Design review of the part shown in the three views and the two pictorial views. Dimensions are in mm from the part's minimum x, y and z. Round coordinates to 2 decimals unless told otherwise and drop trailing zeros. Loops run counter-clockwise (first coordinate to the right, second up) from the corner with the lowest first, then second, coordinate; pieces in that order, holes last. Notation, with made-up numbers: (59.5, -4.5) -> (107.5, -4.5) arc R24 ccw to (107.5, 20.5) -> close; hole circle Ø8 at (14.25, 87). An arc over 180 degrees is marked (long way). Use a Markdown table: item, result. Add a question column.
1) Consider section A-A on x = 2.85. Give the boundary of the cut face in (y, z).
2) Consider section B-B on z = 15.5. Give the boundary of the cut face in (x, y), plus the area to 3 significant figures.
3) Wall thickness on probe 1 along Z at (x, y) = (2, 4.65); probe 2 along Y at (x, z) = (2.95, 10.5); probe 3 along Y at (x, z) = (4.95, 31): over which ranges is each line inside the solid? List them lowest first.
4) Consider section C-C on y = 3.75. Give the boundary of the cut face in (x, z).
5) Mouldability with a two-part tool opening along Z and no side actions: class the marked faces 1, 2 and 3 as released by +Z, released by -Z, zero draft, split by the parting line, or undercut.
6) Insertion check: pin 1 (0.6 mm diameter, centred on x = 2.5, z = 16, fed in from -Y); pin 2 (3 mm diameter, centred on x = 4.5, z = 17, fed in from +Y); pin 3 (2 mm diameter, centred on x = 1.5, z = 30.5, fed in from -Y). Each pin has a flat end and moves straight along its axis. Give the tip position at first contact, or say it passes through.
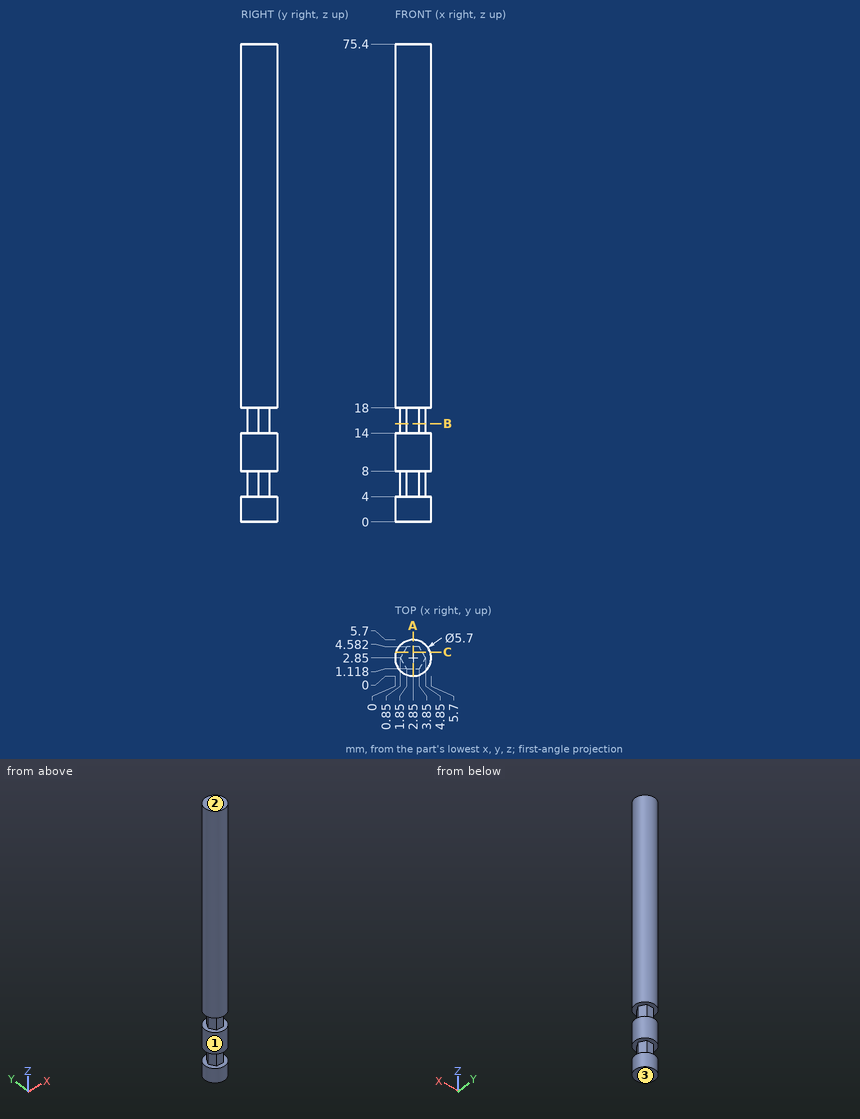
Result set:
| question | item | result |
|---|---|---|
| 1 | outline | (0, 0) -> (5.7, 0) -> (5.7, 4) -> (4.58, 4) -> (4.58, 8) -> (5.7, 8) -> (5.7, 14) -> (4.58, 14) -> (4.58, 18) -> (5.7, 18) -> (5.7, 75.4) -> (0, 75.4) -> (0, 18) -> (1.12, 18) -> (1.12, 14) -> (0, 14) -> (0, 8) -> (1.12, 8) -> (1.12, 4) -> (0, 4) -> close |
| 2 | outline | (0.85, 2.85) -> (1.85, 1.12) -> (3.85, 1.12) -> (4.85, 2.85) -> (3.85, 4.58) -> (1.85, 4.58) -> close |
| 2 | area | 10.4 mm2 |
| 3 | probe 1 | 0 to 4, 8 to 14, 18 to 75.4 |
| 3 | probe 2 | 0 to 5.7 |
| 3 | probe 3 | 0.92 to 4.78 |
| 4 | outline | (0.15, 0) -> (5.55, 0) -> (5.55, 4) -> (4.33, 4) -> (4.33, 8) -> (5.55, 8) -> (5.55, 14) -> (4.33, 14) -> (4.33, 18) -> (5.55, 18) -> (5.55, 75.4) -> (0.15, 75.4) -> (0.15, 18) -> (1.37, 18) -> (1.37, 14) -> (0.15, 14) -> (0.15, 8) -> (1.37, 8) -> (1.37, 4) -> (0.15, 4) -> close |
| 5 | face 1 | zero draft |
| 5 | face 2 | released by +Z |
| 5 | face 3 | released by -Z |
| 6 | pin 1 | y = 1.12 |
| 6 | pin 2 | y = 5.65 |
| 6 | pin 3 | y = 0.02 |
